Part print with two shaded views. Sizes in mm from the minimum x, y, z corner. Give positions to 0.01 mm unless a question says otherwise; leave off trailing zeros. Write each loop counter-clockwise with the first axis right and the second up, starting at its lowest first coordinate (ties: lowest second). Pieces come first, ordered by that corner, then holes. Notation, with made-up numbers: (26, -27) - (36, -27) arc R18 cw to (36, -16) - close; hole circle Ø9 at (-2.75, 8.25). An arc over 180 degrees is marked (long way). One line per item, written item: value. Start each with the question number.
(1) Cut at C-C, the plane y = 6. List the corners of the cut face in (x, z), and give its area (3 significant figures).
(2) Cut at B-B, the plane z = 12. List the corners of the cut face in (x, y), and give its area (3 significant figures).
(3) Probe L1, parallel to Y at x = 22, z = 40.5; L2, parallel to Y at x = 18, z = 24; L3, parallel to X at y = 30.5, z = 4.5. List the from-to ranges inside material, lowest first.
(4) Drop flat-ended pins along their axis: P1, Ø8, axis at x = 7, z = 9.5, coming from the -Y side; P2, Ø8, axis at x = 8.5, z = 54.5, coming from the +Y side; P3, Ø12, axis at x = 42.5, z = 19, coming from the +Y side; P4, Ø3, axis at y = 43.5, z = 14, coming from the -X side. Give the stop position or say it passes through.
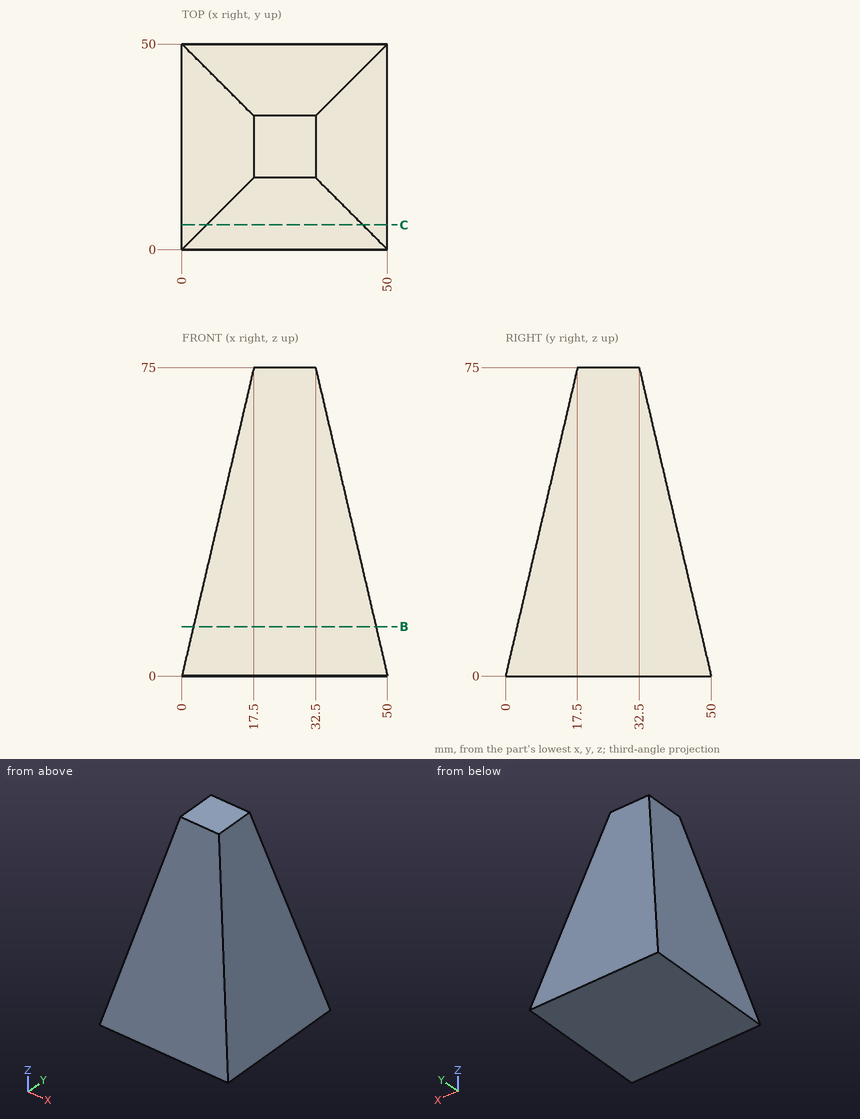
Answers follow:
1. outline: (0, 0) - (50, 0) - (44, 25.71) - (6, 25.71) - close
1. area: 1,130 mm²
2. outline: (2.8, 2.8) - (47.2, 2.8) - (47.2, 47.2) - (2.8, 47.2) - close
2. area: 1,970 mm²
3. L1: y = 9.45 to 40.55
3. L2: y = 5.6 to 44.4
3. L3: x = 1.05 to 48.95
4. P1: stops at y = 1.28
4. P2: passes through
4. P3: stops at y = 46.97
4. P4: stops at x = 2.92
